Here's how the part is built. I have some questions about the finished solid (model axes, mm). A direction names the side the tool comes from. Give positions to 0.01 mm unless a question says otherwise; leave off trailing zeros. Write each loop counter-clockwise with the first axis right and the second up, starting at its lowest first coordinate (ties: lowest second). Pieces come first, ordered by that corner, then holes. Notation, with made-up numbers: M -5.5,1.25 L 52.5,1.25 A30 cw 52.5,29.25 Z; hole C 29.5,9 d8. An arc over 180 degrees is marked long. Answer as CSV lines item,"result". Start each with the question number.
Q1. Suppose I cut it at B-B (x = 4). Write out the boundary of the cut face in (y, z), then the cut area to 3 significant figures.
Q2. For pin 1 (10 mm diameter, centred on x = 10.5, y = 34.5, fed in from +Z), with a flat end and sliding along its axis, tell me the tip position at first contact or that it passes through.
Q3. Suppose I cut it at D-D (x = -20.25). Write out the boundary of the cut face in (y, z).
Q4. Suppose I cut it at A-A (y = 10.5). Write out the boundary of the cut face in (x, z), then the cut area to 3 significant figures.
Q5. If I drill on line 1 along X through (y, z) = (-9.5, 6); line 2 along Y through (x, z) = (-20.25, 44); line 3 along Y through (x, z) = (12.5, 43.5), over which ranges is the centre line in solid material (lowest first)?
Q6. On a 3-axis mill with a long thin cutter (end or side, diameter ignored), from which of +Z, -Z, +X, -X, +Y, -Y can I reach the whole of each face in a straight line? I mean faces 1 (the cylindrical face through (17.15, -36.89, 28.59)), 2 (the flat face through (0, 45, 29)). Say none if no direction works.
Q7. Suppose I cut it at C-C (z = 11). Write out the boundary of the cut face in (x, y), then the cut area to 3 significant figures.
Q8. Thinking about a two-plate mould opening in Y: for faces 3 (the cylindrical face through (-24.1, 44.14, 28.59)), 4 (the flat face through (0, -42, 29)), 5 (the cylindrical face through (24.1, -44.14, 28.59)), 6 (the flat face through (-22.3, 6.9, 0)), which applies, +Y half, -Y half, draft (parallel to the pull), parting line (faces both ways), or undercut?
```python
from build123d import *

# Parameters (mm, degrees)
F0_R     = 2.25
F1_DEPTH = 58


with BuildPart() as f1:
    # F0 (on Top) → F1 (new body)
    with BuildSketch(Plane.XY):
        with BuildLine():
            Line((-22, -45), (22, -45))
            ThreePointArc((22, -45), (24.12132, -44.12132), (25, -42))
            Line((25, -42), (25, 42))
            ThreePointArc((25, 42), (24.12132, 44.12132), (22, 45))
            Line((22, 45), (-22, 45))
            ThreePointArc((-22, 45), (-24.12132, 44.12132), (-25, 42))
            Line((-25, 42), (-25, -42))
            ThreePointArc((-25, -42), (-24.12132, -44.12132), (-22, -45))
        make_face()
        with Locations((-20.25, -38)):
            Circle(F0_R, mode=Mode.SUBTRACT)
        with Locations((20.25, -38)):
            Circle(F0_R, mode=Mode.SUBTRACT)
        with Locations((-20.25, 38)):
            Circle(F0_R, mode=Mode.SUBTRACT)
        with BuildLine():
            ThreePointArc((22, -25), (17.020815, -37.020815), (5, -42))
            Line((5, -42), (-5, -42))
            ThreePointArc((-5, -42), (-17.020815, -37.020815), (-22, -25))
            Line((-22, -25), (-22, 25))
            ThreePointArc((-22, 25), (-17.020815, 37.020815), (-5, 42))
            Line((-5, 42), (5, 42))
            ThreePointArc((5, 42), (17.020815, 37.020815), (22, 25))
            Line((22, 25), (22, -25))
        make_face(mode=Mode.SUBTRACT)
        with Locations((20.25, 38)):
            Circle(F0_R, mode=Mode.SUBTRACT)
    extrude(amount=F1_DEPTH)


solid = f1.part
```
Resolved:
1,outline,"M -45,0 L -42,0 L -42,58 L -45,58 Z; M 42,0 L 45,0 L 45,58 L 42,58 Z"
1,area,"348 mm^2"
2,pin 1,"through"
3,outline,"M -45,0 L -40.25,0 L -40.25,58 L -45,58 Z; M -35.75,0 L -32.51,0 L -32.51,58 L -35.75,58 Z; M 32.51,0 L 35.75,0 L 35.75,58 L 32.51,58 Z; M 40.25,0 L 45,0 L 45,58 L 40.25,58 Z"
4,outline,"M -25,0 L -22,0 L -22,58 L -25,58 Z; M 22,0 L 25,0 L 25,58 L 22,58 Z"
4,area,"348 mm^2"
5,line 1,"-25 to -22, 22 to 25"
5,line 2,"-45 to -40.25, -35.75 to -32.51, 32.51 to 35.75, 40.25 to 45"
5,line 3,"-45 to -40.26, 40.26 to 45"
6,face 1,"+Z, -Z"
6,face 2,"+Z, -Z, +X, -X, +Y"
7,outline,"M -25,-42 A3 ccw -22,-45 L 22,-45 A3 ccw 25,-42 L 25,42 A3 ccw 22,45 L -22,45 A3 ccw -25,42 Z; hole C -20.25,-38 d4.5; hole C -20.25,38 d4.5; hole M -22,-25 A17 ccw -5,-42 L 5,-42 A17 ccw 22,-25 L 22,25 A17 ccw 5,42 L -5,42 A17 ccw -22,25 Z; hole C 20.25,-38 d4.5; hole C 20.25,38 d4.5"
7,area,"981 mm^2"
8,face 3,"+Y half"
8,face 4,"undercut"
8,face 5,"-Y half"
8,face 6,"draft"
